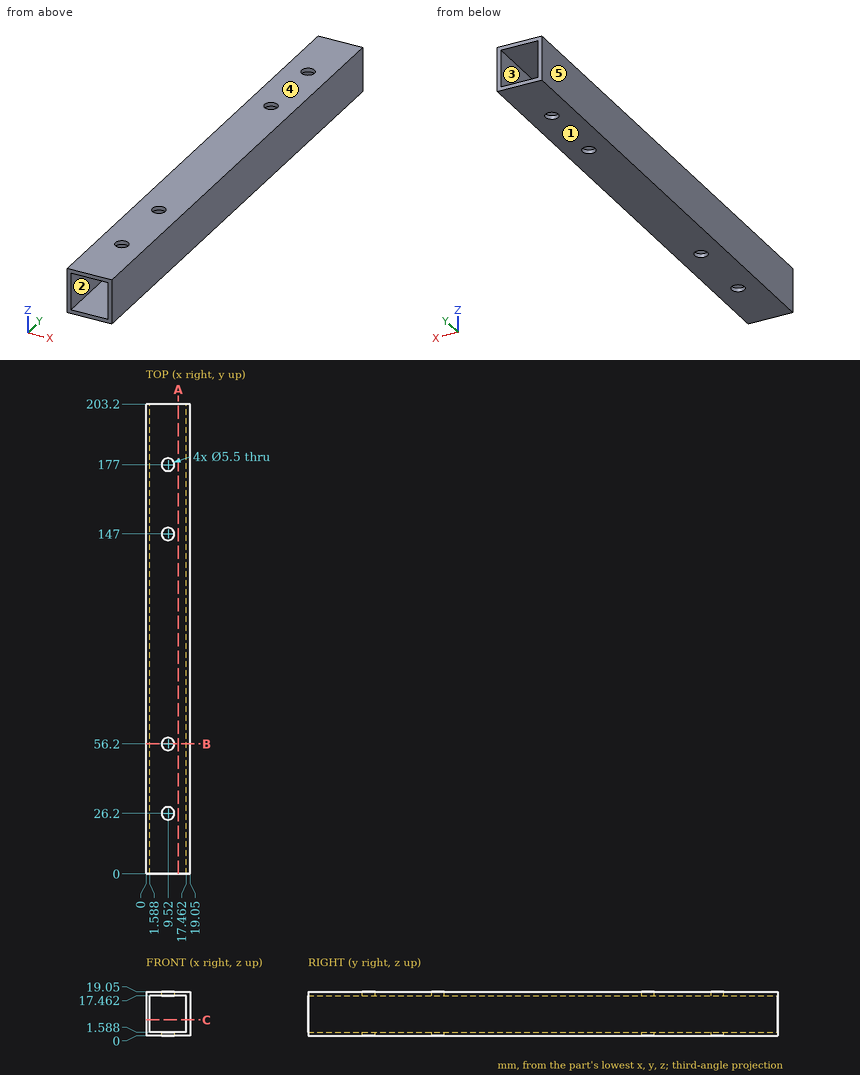
Study the drawing (mm; zero at the part's minimum x, y, z) and answer. A direction names the side the tool comes from. Coordinates: 2 decimals unless noted, no trailing zeros. Order: outer loops, then holes, each group sorted by start corner. A loop starts at its lowest first (then second) coordinate and runs counter-clockwise, first axis right, second up. Notation, with made-up numbers: M -23.5,81.25 L -4.5,81.25 A20 ccw -4.5,98.25 Z; hole C 64.25,76 d2. An arc over 180 degrees is marked long. Answer as a JSON object with one key per item and string values. Group by question number.
1. A flat-ended cylindrical pin translates along its axis: P1, Ø4.5, axis at x = 9.52, y = 56.2, coming from the +Z side. Find the tip coordinate at first contact, or state that the pin passes through.
2. Section B-B on y = 56.2 is taken. Write down the section's boundary in (x, z).
3. Determine the mould class of the marked faces 3, 4 and 5 for opening direction Z: released by +Z, released by -Z, zero draft, split by the parting line, or undercut.
4. A tool of negligible diameter and unlimited length cuts with its end or side. For the marked faces 1 and 2, from which of +Z, -Z, +X, -X, +Y, -Y can it reach the whole face along a straight path? Write none if from no direction.
5. Section A-A on x = 14 is taken. Write down the section's boundary in (y, z).
6. Straight lines are drawn through the part: line 1 (Y direction, x = 9.52, z = 18.45); line 2 (Z direction, x = 3, y = 153.5). For each, find the intervals that lie inside material, in ascending order.
7. Section C-C on z = 7 is taken. Write down the section's boundary in (x, y).
Values follow:
{
 "1": {"P1": "through"},
 "2": {"outline": "M 0,0 L 6.77,0 L 6.77,1.59 L 1.59,1.59 L 1.59,17.46 L 6.77,17.46 L 6.77,19.05 L 0,19.05 Z; M 12.27,0 L 19.05,0 L 19.05,19.05 L 12.27,19.05 L 12.27,17.46 L 17.46,17.46 L 17.46,1.59 L 12.27,1.59 Z"},
 "3": {"face 3": "undercut", "face 4": "released by +Z", "face 5": "zero draft"},
 "4": {"face 1": "-Z, +X, -X, +Y, -Y", "face 2": "+Y, -Y"},
 "5": {"outline": "M 0,0 L 203.2,0 L 203.2,1.59 L 0,1.59 Z; M 0,17.46 L 203.2,17.46 L 203.2,19.05 L 0,19.05 Z"},
 "6": {"line 1": "0 to 23.45, 28.95 to 53.45, 58.95 to 144.25, 149.75 to 174.25, 179.75 to 203.2", "line 2": "0 to 1.59, 17.46 to 19.05"},
 "7": {"outline": "M 0,0 L 1.59,0 L 1.59,203.2 L 0,203.2 Z; M 17.46,0 L 19.05,0 L 19.05,203.2 L 17.46,203.2 Z"}
}
